Can you work these out from the model? Positions are in its coordinate system, mm. A direction names the side the tool comes from. Coordinates: 2 decimals unless noted, no trailing zeros. Write each loop counter-clockwise with the first axis right and the second up, starting at its lowest first coordinate (ties: lowest second). Pieces come first, ordered by that corner, then holes. Notation, with made-up numbers: (45, 85.25) - (78, 85.25) arc R24 ccw to (78, 117.25) - close; hole circle Ø11 at (50.25, 29.5). An arc over 180 degrees is marked (long way). Write each question's results on one line, items separated by ' | '. Start each with the question number.
Autodesk Inventor part; units mm, degrees
ref_plane "YZ Plane" through (0, 0, 0) normal (1, 0, 0) x (0, 1, 0)
ref_plane "XZ Plane" through (0, 0, 0) normal (0, 1, 0) x (-1, 0, 0)
ref_plane "XY Plane" through (0, 0, 0) normal (0, 0, 1) x (1, 0, 0)
sketch "Sketch2: RFID holder" plane through (0, 0, 0) normal (1, 0, 0) x (0, 0, -1)
  circle A0 centre (-28.125, 0) radius 16.25
  circle A1 centre (-28.125, 0) radius 22
  circle A2 centre (-28.125, 0) radius 24.625
  circle A3 centre (-28.125, 0) radius 25.375
  line L0 (-28.125, 1.5) -> (0, 1.5)
  line L1 (-28.125, -1.5) -> (0, -1.5)
  line L2 (0, -13.4) -> (0, 13.4)
  line L3 (0, -13.4) -> (-3.5, -13.4)
  line L4 (0, 13.4) -> (-3.5, 13.4)
  line L5 (-3.5, 13.4) -> (-3.5, -13.4)
  line L6 (-28.125, 1.5) -> (-28.125, -1.5) construction
  line L7 (-2.75, 13.4) -> (-2.75, -13.4) construction
  line L8 (-1, 13.4) -> (-1, -13.4)
  line L9 (-3.5, -6.1237) -> (0, -6.1237)
  point P0 (-2.7944, -1.5)
  point P1 (-2.7944, 1.5)
  point P2 (0, 0)
  point P3 (-6.1762, -1.5)
  point P4 (-6.1762, 1.5)
  point P5 (-3.5457, -1.5)
  point P6 (-3.5457, 1.5)
  point P7 (-3.5, -1.5)
  point P8 (-3.5, 1.5)
  point P9 (-3.5, 0)
  point P10 (0, 0)
  point P11 (-3.5, 6.1237)
  point P12 (-3.5, -6.1237)
  point P13 (-1, -1.5)
  point P14 (-1, 1.5)
  dimension "d48" = 50.75
  dimension "RFID_coil_ID" = 44
  dimension "RFID_coil_OD" = 49.25
  dimension "d7" = 0.75
  dimension "d49" = 3
  dimension "d54" = 1.5
  dimension "d57" = 0.75
  dimension "d58" = 26.8
  dimension "d59" = 3.5
  dimension "d60" = 32.5
  dimension "dist_for_RFID_wire" = 2.5
sketch "Sketch8: M3 through hole" plane through (0, 0, 0) normal (1, 0, 0) x (0, 1, 0)
  line L0 (20.4, 7) -> (13.4, 7)
  line L1 (13.4, 7) -> (13.4, 0)
  line L2 (13.4, 0) -> (20.4, 0)
  line L3 (20.4, 0) -> (20.4, 7)
  circle A0 centre (16.9, 3.5) radius 1.85
  circle A1 centre (0, 28.125) radius 25.375
  line L4 (13.4, 3.5) -> (-13.4, 3.5)
  line L5 (13.4, 0) -> (13.4, 3.5) construction
  point P0 (0, 0)
  point P1 (20.4, 3.5)
  point P2 (16.9, 7)
  point P3 (6.1237, 3.5)
  point P4 (14.0579, 7)
  dimension "d63" = 3.7
  dimension "d66" = 7
  dimension "d67" = 7
extrude "Ex2: RFID holder base" add sketch "Sketch2: RFID holder" against normal blind 3.25 contours A0 L0 A1 L1 | A0 L1 A1 L0 | L0 A2 L1 A1 | A1 L1 A2 L0 | L0 L5 A2 | A2 L1 L5 A3 L0 | A2 L5 L1 | L5 L0 A3 L1 | L5 A3 L0 | L1 A3 L5 | L0 L8 L1 A3 | A3 L5 L4 L8 L0 | L1 L8 L9 A3 | L9 L8 L3 L5 | L8 L4 L2 L0 | L0 L2 L1 L8 | L1 L2 L9 L8 | L9 L2 L3 L8
extrude "Ex3: RFID inset" cut sketch "Sketch2: RFID holder" against normal blind 2.25 contours L0 A2 L1 A1 | A1 L1 A2 L0
extrude "Ex4: RFID wire cutout" [suppressed]
extrude "Ex: M3 through hole" add sketch "Sketch8: M3 through hole" against normal up to surface (3.25 mm away) contours L3 L2 L1 A1 L0 | L1 L4 A1
properties part number "RFID_holder_coil_01" material "PLA Black"
Q1. I'm going to push flat-ended pins straight in: pin 1 Ø2 at (y, z) = (-4.5, 48) entering from +X; pin 2 Ø1.6 at (x, z) = (-1, 3.5) entering from +Y; pin 3 Ø1.6 at (x, z) = (-2.5, 1.5) entering from -Y; pin 4 Ø1.6 at (x, y) = (-2, -8.5) entering from +Z. Where does each tip first touch, or does it pass through?
Q2. Thinking about a two-plate mould opening in Y: for faces 1 (the face through (-1.11, 7.4, 4.64)), 2 (the face through (-2, 20.4, 3)), 3 (the face through (-1.6, 0.71, 44.36)), 4 (the face through (0, 2, 3)), which applies, pulls with the +Y half, pulls with the -Y half, needs draft (parallel to the pull), parting line crosses it, or undercut?
Q3. For faces 5 (the face through (-2, -13.4, 2)), 6 (the face through (-1.109, -8.426, 7.803)), 7 (the face through (0, -15, 36)), which set-ups out of +Z, -Z, +X, -X, +Y, -Y let a thin tool reach every point of the face, with its end or its side?
Q4. If we section it at D-D (y = 16.9): Please give me the cut outline in (x, z), then the cut area to 3 significant figures.
Q5. If we section it at A-A (y = 0): Please give me the cut outline in (x, z) (3 decimals).
Q6. If we section it at C-C (z = 21): Please give me the cut outline in (x, y), then the cut area to 3 significant figures.
Q7. I need wall thicknesses on line 1 along Z through (x, y) = (-1.95, 0) (3 decimals); line 2 along Y through (x, z) = (-0.55, 29); line 3 along Y through (x, z) = (-2.05, 31.5). Which ranges of each line are inside material? Lowest first, please. Write a range as from..to.
Q8. If we section it at B-B (x = -0.7): Please give me the cut outline in (y, z) (3 decimals), then the cut area to 3 significant figures.
Answer list:
1) pin 1: stops at x = 0 | pin 2: stops at y = 20.4 | pin 3: stops at y = -13.4 | pin 4: stops at z = 52.3
2) face 1: undercut | face 2: pulls with the +Y half | face 3: undercut | face 4: needs draft
3) face 5: -Z, +X, -X, -Y | face 6: +X | face 7: +Z, -Z, +X, +Y, -Y
4) outline: (-3.25, 0) - (0, 0) - (0, 1.65) - (-3.25, 1.65) - close; (-3.25, 5.35) - (0, 5.35) - (0, 7) - (-3.25, 7) - close; (-3.25, 9.2) - (0, 9.2) - (0, 10.21) - (-2.25, 10.21) - (-2.25, 14.04) - (0, 14.04) - (0, 42.21) - (-2.25, 42.21) - (-2.25, 46.04) - (0, 46.04) - (0, 47.05) - (-3.25, 47.05) - close | area: 117 mm2
5) outline: (-3.25, 0) - (0, 0) - (0, 3.5) - (-2.25, 3.5) - (-2.25, 6.125) - (0, 6.125) - (0, 11.875) - (-3.25, 11.875) - close; (-3.25, 44.375) - (0, 44.375) - (0, 50.125) - (-2.25, 50.125) - (-2.25, 52.75) - (0, 52.75) - (0, 53.5) - (-3.25, 53.5) - close
6) outline: (-3.25, -24.35) - (0, -24.35) - (0, -23.57) - (-2.25, -23.57) - (-2.25, -20.81) - (0, -20.81) - (0, -14.6) - (-3.25, -14.6) - close; (-3.25, 14.6) - (0, 14.6) - (0, 20.81) - (-2.25, 20.81) - (-2.25, 23.57) - (0, 23.57) - (0, 24.35) - (-3.25, 24.35) - close | area: 51.0 mm2
7) line 1: z = 0..3.5, 6.125..11.875, 44.375..50.125, 52.75..53.5 | line 2: y = -25.36..-24.61, -21.98..-16.23, 16.23..21.98, 24.61..25.36 | line 3: y = -25.15..-24.39, -21.74..-15.9, 15.9..21.74, 24.39..25.15
8) outline: circle Ø44 at (0, 28.125); (-13.4, 0) - (20.4, 0) - (20.4, 7) - (14.058, 7) arc R25.375 ccw (long way) to (-6.124, 3.5) - (-13.4, 3.5) - close; hole circle Ø49.25 at (0, 28.125); hole circle Ø32.5 at (0, 28.125); hole circle Ø3.7 at (16.9, 3.5) | area: 944 mm2
